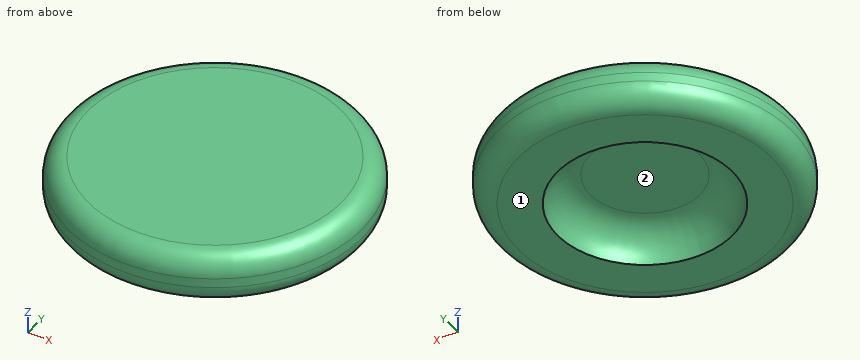
```python
from build123d import *

# Parameters (mm, degrees)
F0_R     = 22.5
F0_R_2   = 13.3867529453
F1_DEPTH = 7.7
F2_R     = 3.1384776311
F3_DEPTH = 3


# Not quite as in the source:
# - a fillet or chamfer that OpenCascade refuses, or shapes differently, is made with other operations: its cross-section is extruded or revolved along the edge and cut away or added


with BuildPart() as f1:
    # F0 (on Top) → F1 (new body)
    with BuildSketch(Plane.XY):
        with Locations((-30.7742264122, 10.8950231224)):
            Circle(F0_R)
        with Locations((-30.7742264122, 10.8950231224)):
            Circle(F0_R_2, mode=Mode.SUBTRACT)
    extrude(amount=-F1_DEPTH)

    # F2
    f2_edges = [f1.edges().sort_by_distance(p)[0] for p in [
        (-8.274226, 10.895023, -3.85),
        (-53.274226, 10.895023, 0),
        (-53.274226, 10.895023, -7.7),
    ]]
    fillet(f2_edges, radius=F2_R)

    # F0 (on Top) → F3 (join)
    with BuildSketch(Plane.XY):
        with Locations((-30.7742264122, 10.8950231224)):
            Circle(F0_R_2)
    extrude(amount=-F3_DEPTH)

    # F4: fillet of radius 5 on 1 edges, made by hand

    # F4_s1 → F4_t2 (revolve)
    with BuildSketch(Plane.XZ.offset(-10.8950231224)):
        with BuildLine():
            ThreePointArc((-17.3874734669, -7.7), (-18.9506380521, -4.3599450554), (-22.3784653523, -3))
            Line((-22.3784653523, -3), (-17.3874734669, -3))
            Line((-17.3874734669, -3), (-17.3874734669, -7.7))
        make_face()
    revolve(axis=Axis((-30.7742264122, 10.8950231224, -3), (0, 0, 1)))


solid = f1.part
```
Geometry check sheet. Reference: the model listing, model coordinates, mm. Face numbers are marked on the shaded views. Round coordinates to 2 decimals unless told otherwise and drop trailing zeros. Loops run counter-clockwise (first coordinate to the right, second up) from the corner with the lowest first, then second, coordinate; pieces in that order, holes last. Notation, with made-up numbers: (48, -10) - (94, -10) arc R17 ccw to (94, 22) - close; hole circle Ø11 at (28, 76). An arc over 180 degrees is marked (long way). Write item = value, one per line. Start each with the question number.
1. Mould release check, pull along X, two halves, no side actions. Record for the marked faces 1 and 2: released by +X, released by -X, zero draft, split by the parting line, or undercut.
2. Thickness scan on line 1 (Y direction, x = -41, z = -4.25); line 2 (Y direction, x = -31.5, z = -5.5); line 3 (Z direction, x = -33.5, y = 13). Record the ranges inside material, lowest first.
3. Section check B-B on z = -1. Enter the section's corners in (x, y).
4. Section check A-A on z = -5.25. Enter the section's corners in (x, y), then the cut area to 3 significant figures.
5. Depth check by flat-ended pin: pin 1 (1.5 mm diameter, centred on x = -39.5, z = -2, fed in from +Y); pin 2 (2 mm diameter, centred on x = -19.5, z = -5.5, fed in from -Y); pin 3 (1.5 mm diameter, centred on y = 23, z = -2, fed in from +X). Enter the tip coordinate at first touch or a pass-through.
Working result:
q1.face_1 = zero draft
q1.face_2 = undercut
q2.line_1 = -9.15 to 5.2, 16.59 to 30.94
q2.line_2 = -11.45 to -1.81, 23.6 to 33.24
q2.line_3 = -3 to 0
q3.outline = circle Ø43.32 at (-30.77, 10.9)
q4.outline = circle Ø44.85 at (-30.77, 10.9); hole circle Ø25.14 at (-30.77, 10.9)
q4.area = 1,080 mm^2
q5.pin_1 = 31.8
q5.pin_2 = -9.03
q5.pin_3 = -11.52
